from build123d import *

# Parameters (mm, degrees)
SKETCH_1_R               = 15
EXTRUDE_1_DEPTH          = 10
CUT_EXTRUDE_1_DEPTH      = 49.218253805
CUT_EXTRUDE_1_DEPTH_BACK = 49.218253805
SKETCH_2_R               = 1.5
CUT_EXTRUDE_2_DEPTH      = 2
SKETCH_4_R               = 1.5
CUT_EXTRUDE_3_DEPTH      = 3


with BuildPart() as part:
    # 草图1 → 凸台-拉伸1 (new body)
    with BuildSketch(Plane.XY):
        Polygon((-25, -20), (-25, -15), (-20, -12.113248654), (-20, 12.113248654), (-25, 15), (-25, 20), (25, 20), (25, 15), (20, 12.113248654), (20, -12.113248654), (25, -15), (25, -20), align=None)
        Circle(SKETCH_1_R, mode=Mode.SUBTRACT)
    extrude(amount=EXTRUDE_1_DEPTH)

    # 草图2 → 切除-拉伸1 (cut, two sides: drawn at the far end of the back side and taken through both)
    with BuildSketch(Plane(origin=(0, 20, 0), x_dir=(1, 0, 0), z_dir=(0, 1, 0)).offset(-CUT_EXTRUDE_1_DEPTH_BACK)):
        with Locations((-22, -5)):
            Circle(SKETCH_2_R)
        with Locations((22, -5)):
            Circle(SKETCH_2_R)
    extrude(amount=CUT_EXTRUDE_1_DEPTH + CUT_EXTRUDE_1_DEPTH_BACK, mode=Mode.SUBTRACT)

    # 草图3 → 切除-拉伸2 (cut)
    with BuildSketch(Plane(origin=(0, 20, 0), x_dir=(1, 0, 0), z_dir=(0, 1, 0))):
        with BuildLine():
            Line((-16.5, -2), (16.5, -2))
            ThreePointArc((16.5, -2), (19.5, -5), (16.5, -8))
            Line((16.5, -8), (-16.5, -8))
            ThreePointArc((-16.5, -8), (-19.5, -5), (-16.5, -2))
        make_face()
    cut_extrude_2 = extrude(amount=-CUT_EXTRUDE_2_DEPTH, mode=Mode.SUBTRACT)

    # 草图4 → 切除-拉伸3 (cut)
    with BuildSketch(Plane(origin=(0, 18, 0), x_dir=(1, 0, 0), z_dir=(0, 1, 0))):
        with Locations(Location((-16.5, -5, 0), (0, 0, 180))):
            Circle(SKETCH_4_R)
        with Locations((16.5, -5)):
            Circle(SKETCH_4_R)
    cut_extrude_3 = extrude(amount=-CUT_EXTRUDE_3_DEPTH, mode=Mode.SUBTRACT)

    # 镜向1: 切除-拉伸2, 切除-拉伸3 across plane
    add(cut_extrude_2.mirror(Plane.ZX), mode=Mode.SUBTRACT)
    add(cut_extrude_3.mirror(Plane.ZX), mode=Mode.SUBTRACT)


solid = part.part
Read the model definition and answer for the solid it produces. Units are mm, in the model's axes. A direction names the side the tool comes from. Round coordinates to 2 decimals unless told otherwise and drop trailing zeros. Order: outer loops, then holes, each group sorted by start corner. A loop starts at its lowest first (then second) coordinate and runs counter-clockwise, first axis right, second up.
1) The part is cut by section B-B on z = 1.25. Write down the section's boundary in (x, y).
2) The part is cut by section A-A on y = -9. Write down the section's boundary in (x, z).
3) For faces 4 (the face through (0, 19, 2)), 5 (the face through (-19.5, -19, 5.1)), 6 (the face through (-25, 17, 5)), determine the directions among +Z, -Z, +X, -X, +Y, -Y from which every point of the face is accessible in a straight line to the end or side of a thin tool.
4) Straight lines are drawn through the part: L1, parallel to Z at x = 22, y = -17; L2, parallel to Y at x = 0, z = 4.5; L3, parallel to Y at x = 3, z = 4.25. For each, find the intervals that lie inside material, in ascending order.
5) The part is cut by section C-C on x = 9. Write down the section's boundary in (y, z), plus the area to 3 significant figures.
6) The part is cut by section D-D on x = 22. Write down the section's boundary in (y, z).
7) The mould has two halves that part along X. Classify faces 1 (the face through (-23.58, 14.18, 3.82)), 2 (the face through (17, 0, 0)), 3 (the face through (-20.57, 16.99, 4.55)): released by +X, released by -X, zero draft, split by the parting line, or undercut.
8) Flat-ended cylindrical pins translate along their axes: pin 1 (5 mm diameter, centred on x = 16.5, z = 5, fed in from +Y); pin 2 (2 mm diameter, centred on y = 12, z = 6.5, fed in from +X); pin 3 (2.5 mm diameter, centred on x = -16.5, z = 5, fed in from -Y); pin 4 (2.5 mm diameter, centred on x = -22, z = 5, fed in from +Y). Find the tip coordinate at first contact, or state that the pin passes through.
Resolved:
1. outline: (-25, -20) - (25, -20) - (25, -15) - (20, -12.11) - (20, 12.11) - (25, 15) - (25, 20) - (-25, 20) - (-25, 15) - (-20, 12.11) - (-20, -12.11) - (-25, -15) - close; hole circle Ø30 at (0, 0)
2. outline: (-20, 0) - (-12, 0) - (-12, 10) - (-20, 10) - close; (12, 0) - (20, 0) - (20, 10) - (12, 10) - close
3. face 4: +Y
3. face 5: -Y
3. face 6: +Z, -Z, -X, +Y, -Y
4. L1: z = 0 to 3.5, 6.5 to 10
4. L2: y = -18 to -15, 15 to 18
4. L3: y = -18 to -14.7, 14.7 to 18
5. outline: (-20, 0) - (-12, 0) - (-12, 10) - (-20, 10) - (-20, 8) - (-18, 8) - (-18, 2) - (-20, 2) - close; (12, 0) - (20, 0) - (20, 2) - (18, 2) - (18, 8) - (20, 8) - (20, 10) - (12, 10) - close
5. area: 136 mm2
6. outline: (-20, 0) - (-13.27, 0) - (-13.27, 3.5) - (-20, 3.5) - close; (-20, 6.5) - (-13.27, 6.5) - (-13.27, 10) - (-20, 10) - close; (13.27, 0) - (20, 0) - (20, 3.5) - (13.27, 3.5) - close; (13.27, 6.5) - (20, 6.5) - (20, 10) - (13.27, 10) - close
7. face 1: released by -X
7. face 2: zero draft
7. face 3: undercut
8. pin 1: stops at y = 18
8. pin 2: stops at x = 21.54
8. pin 3: stops at y = -15
8. pin 4: passes through
